Geometry: final body of the model. Coordinates: model frame, mm. A direction names the side the tool comes from. Round coordinates to 2 decimals unless told otherwise and drop trailing zeros. Loops run counter-clockwise (first coordinate to the right, second up) from the corner with the lowest first, then second, coordinate; pieces in that order, holes last. Notation, with made-up numbers: (-13.5, -1.75) -> (14.5, -1.75) arc R20 cw to (14.5, 35.25) -> close; hole circle Ø9 at (-18, -31.5). An arc over 180 degrees is marked (long way). Answer in a Markdown table with one row per item.
```python
from build123d import *

# Parameters (mm, degrees)
SKETCH_1_W          = 60
SKETCH_1_H          = 63.5
SKETCH_1_R          = 12
SKETCH_1_R_2        = 4
EXTRUDE_1_DEPTH     = 10
CHAMFER_1_SIZE      = 0.25
SKETCH_2_W          = 60
SKETCH_2_H          = 5
EXTRUDE_2_DEPTH     = 60
MM_START            = -31.75
MM_1_DEPTH          = 5
SKETCH_8_R          = 4.75
SKETCH_8_R_2        = 4.25
EXTRUDE_3_DEPTH     = 10
EXTRUDE_4_DEPTH     = 20
CHAMFER_4_SIZE      = 2
HOLE_WIZARD_2_D     = 5.4
HOLE_WIZARD_2_DEPTH = 2
HOLE_WIZARD_3_D     = 3.3


# Read off the part's stored shape, not the designer's step: 大小mm 暗销槽口1
with BuildPart() as part:
    # 草图1 → 凸台-拉伸1 (new body)
    with BuildSketch(Plane.XY):
        Rectangle(SKETCH_1_W, SKETCH_1_H)
        Circle(SKETCH_1_R, mode=Mode.SUBTRACT)
        with Locations((20, 0)):
            Circle(SKETCH_1_R_2, mode=Mode.SUBTRACT)
        with Locations(Location((-20, 0, 0), (0, 0, 180))):
            Circle(SKETCH_1_R_2, mode=Mode.SUBTRACT)
    extrude(amount=EXTRUDE_1_DEPTH)

    # 倒角1
    chamfer_1_edges = [part.edges().sort_by_distance(p)[0] for p in [
        (16, 0, 0),
        (-16, 0, 0),
    ]]
    chamfer(chamfer_1_edges, length=CHAMFER_1_SIZE)

    # 草图2 → 凸台-拉伸2 (add)
    with BuildSketch(Plane.XY.offset(10)):
        with Locations((0, -29.25)):
            Rectangle(SKETCH_2_W, SKETCH_2_H)
    extrude(amount=EXTRUDE_2_DEPTH)

    # 大小mm 暗销槽口1 outline → 大小mm 暗销槽口1 (cut)
    with BuildSketch(Plane(origin=(0, 0, 0), x_dir=(1, 0, 0), z_dir=(0, 1, 0)).offset(MM_START)):
        with BuildLine():
            ThreePointArc((23.909259259, -32.749042146), (25.459259259, -34.299042146), (27.009259259, -32.749042146))
            Line((27.009259259, -32.749042146), (27.009259259, -22.749042146))
            ThreePointArc((27.009259259, -22.749042146), (25.459259259, -21.199042146), (23.909259259, -22.749042146))
            Line((23.909259259, -22.749042146), (23.909259259, -32.749042146))
        make_face()
        with BuildLine():
            Line((27.009259259, -67.557471264), (27.009259259, -57.557471264))
            ThreePointArc((27.009259259, -57.557471264), (25.459259259, -56.007471264), (23.909259259, -57.557471264))
            Line((23.909259259, -57.557471264), (23.909259259, -67.557471264))
            ThreePointArc((23.909259259, -67.557471264), (25.459259259, -69.107471264), (27.009259259, -67.557471264))
        make_face()
        with BuildLine():
            Line((-23.909259259, -67.557471264), (-23.909259259, -57.557471264))
            ThreePointArc((-23.909259259, -57.557471264), (-25.459259259, -56.007471264), (-27.009259259, -57.557471264))
            Line((-27.009259259, -57.557471264), (-27.009259259, -67.557471264))
            ThreePointArc((-27.009259259, -67.557471264), (-25.459259259, -69.107471264), (-23.909259259, -67.557471264))
        make_face()
        with BuildLine():
            Line((-23.909259259, -32.749042146), (-23.909259259, -22.749042146))
            ThreePointArc((-23.909259259, -22.749042146), (-25.459259259, -21.199042146), (-27.009259259, -22.749042146))
            Line((-27.009259259, -22.749042146), (-27.009259259, -32.749042146))
            ThreePointArc((-27.009259259, -32.749042146), (-25.459259259, -34.299042146), (-23.909259259, -32.749042146))
        make_face()
    extrude(amount=MM_1_DEPTH, mode=Mode.SUBTRACT)

    # 草图8 → 凸台-拉伸3 (add)
    with BuildSketch(Plane(origin=(0, 0, 0), x_dir=(-1, 0, 0), z_dir=(0, 0, -1))):
        with Locations((20, 0)):
            Circle(SKETCH_8_R)
        with Locations((20, 0)):
            Circle(SKETCH_8_R_2, mode=Mode.SUBTRACT)
    extrude_3 = extrude(amount=EXTRUDE_3_DEPTH)

    # 镜向1: 凸台-拉伸3 across plane
    add(extrude_3.mirror(Plane.ZY))

    # 草图9 → 凸台-拉伸4 (add, symmetric)
    with BuildSketch(Plane.ZY):
        Polygon((0, -31.75), (-10, -41.75), (90, -41.75), (90, -34.25), (70, -34.25), (70, -31.75), align=None)
    extrude(amount=EXTRUDE_4_DEPTH, both=True)

    # 倒角4
    chamfer_4_edges = [part.edges().sort_by_distance(p)[0] for p in [
        (-30, 31.75, 5),
        (30, 31.75, 5),
    ]]
    chamfer(chamfer_4_edges, length=CHAMFER_4_SIZE)

    # 孔2
    with Locations(Plane(origin=(0, -41.75, 0), x_dir=(-1, 0, 0), z_dir=(0, -1, 0))):
        with Locations((-10, -80)):
            hole_wizard_2 = Hole(HOLE_WIZARD_2_D / 2, depth=HOLE_WIZARD_2_DEPTH)

    # 孔3 (through all)
    with Locations(Plane(origin=(0, -41.75, 0), x_dir=(-1, 0, 0), z_dir=(0, -1, 0))):
        with Locations((-10, -80)):
            hole_wizard_3 = Hole(HOLE_WIZARD_3_D / 2)

    # 镜向2: 孔2, 孔3 across plane
    add(hole_wizard_2.mirror(Plane.ZY), mode=Mode.SUBTRACT)
    add(hole_wizard_3.mirror(Plane.ZY), mode=Mode.SUBTRACT)


solid = part.part
```
Item 1: Reachability of faces 1 (the face through (25.425, -29.285, 69.107)), 2 (the face through (9.415, -40.736, 82.636)), 3 (the face through (0, 16, 10)), 4 (the face through (30, -10, 9)), 5 (the face through (-16.868, 2.872, -4.93)) from +Z, -Z, +X, -X, +Y, -Y: full face, straight path, thin tool, end or side. Return the list, or none.
Answer:
| item | result |
|---|---|
| face 1 | +Y, -Y |
| face 2 | -Y |
| face 3 | +Z, +X, -X, +Y |
| face 4 | +Z, -Z, +X, +Y, -Y |
| face 5 | -Z |
Item 2: Cut plane B-B (z = 27.5). Output: boundary loops of the cut face in (x, y).
Answer:
| item | result |
|---|---|
| outline | (-30, -31.75) -> (-27.01, -31.75) -> (-27.01, -26.75) -> (-30, -26.75) -> close; (-23.91, -31.75) -> (-20, -31.75) -> (-20, -41.75) -> (20, -41.75) -> (20, -31.75) -> (23.91, -31.75) -> (23.91, -26.75) -> (-23.91, -26.75) -> close; (27.01, -31.75) -> (30, -31.75) -> (30, -26.75) -> (27.01, -26.75) -> close |
Item 3: Line query: probe 1 along X at (y, z) = (-40.2, 80); probe 2 along X at (y, z) = (-38.35, 80); probe 3 along Z at (x, y) = (8, 16). Output: solid intervals per line, ascending. Write a range as [from, to].
Answer:
| item | result |
|---|---|
| probe 1 | x = [-20, -12.7], [-7.3, 7.3], [12.7, 20] |
| probe 2 | x = [-20, -11.65], [-8.35, 8.35], [11.65, 20] |
| probe 3 | z = [0, 10] |
Item 4: Pin query (flat end, axial travel): pin 1 Ø10 at (x, y) = (18.5, 11.5) entering from +Z; pin 2 Ø5 at (x, z) = (-27, 26.5) entering from -Y; pin 3 Ø22 at (x, z) = (-5.5, 82) entering from +Y; pin 4 Ø7 at (x, y) = (20, 0) entering from +Z. Return the tip coordinate at first contact, or that it passes through.
Answer:
| item | result |
|---|---|
| pin 1 | stops at z = 10 |
| pin 2 | stops at y = -31.75 |
| pin 3 | stops at y = -34.25 |
| pin 4 | passes through |
Item 5: Draft query along Z for faces 6 (the face through (-14, 0, 0)), 7 (the face through (-9.415, -40.736, 82.636)), 8 (the face through (-20, -37, 39)). Return one class per face: pulls with the +Z half, pulls with the -Z half, needs draft (parallel to the pull), parting line crosses it, or undercut.
Answer:
| item | result |
|---|---|
| face 6 | pulls with the -Z half |
| face 7 | undercut |
| face 8 | needs draft |
Item 6: Cut plane A-A (y = 0). Count the separate pieces of the cut face and the enclosed holes in it, then the cut area to 3 significant figures.
Answer:
| item | result |
|---|---|
| separate pieces | 4 |
| enclosed holes | 0 |
| area | 220 mm² |
Item 7: Cut plane C-C (x = 0). Output: boundary loops of the cut face in (y, z).
Answer:
| item | result |
|---|---|
| outline | (-41.75, -10) -> (-31.75, 0) -> (-12, 0) -> (-12, 10) -> (-26.75, 10) -> (-26.75, 70) -> (-34.25, 70) -> (-34.25, 90) -> (-41.75, 90) -> close; (12, 0) -> (31.75, 0) -> (31.75, 10) -> (12, 10) -> close |
Item 8: Cut plane D-D (x = -10). Output: boundary loops of the cut face in (y, z), then the cut area to 3 significant figures.
Answer:
| item | result |
|---|---|
| outline | (-41.75, -10) -> (-31.75, 0) -> (-6.63, 0) -> (-6.63, 10) -> (-26.75, 10) -> (-26.75, 70) -> (-34.25, 70) -> (-34.25, 78.35) -> (-39.75, 78.35) -> (-39.75, 77.3) -> (-41.75, 77.3) -> close; (-41.75, 82.7) -> (-39.75, 82.7) -> (-39.75, 81.65) -> (-34.25, 81.65) -> (-34.25, 90) -> (-41.75, 90) -> close; (6.63, 0) -> (31.75, 0) -> (31.75, 10) -> (6.63, 10) -> close |
| area | 1,670 mm² |
